Source: CAD feature listing. Evaluate the final solid. Frame: model axes, mm. Face numbers are marked on the shaded views. A direction names the side the tool comes from. Give positions to 0.01 mm unless a question says otherwise; leave off trailing zeros. Order: outer loops, then holes, each group sorted by start corner. A loop starts at its lowest first (then second) coordinate and runs counter-clockwise, first axis right, second up. Notation, with made-up numbers: (36.25, 49) - (50.25, 49) arc R23 cw to (50.25, 82) - close; hole circle Ø6 at (75, -37). An arc over 180 degrees is marked (long way). Use CSV: the item, a comma, the result in double quotes.
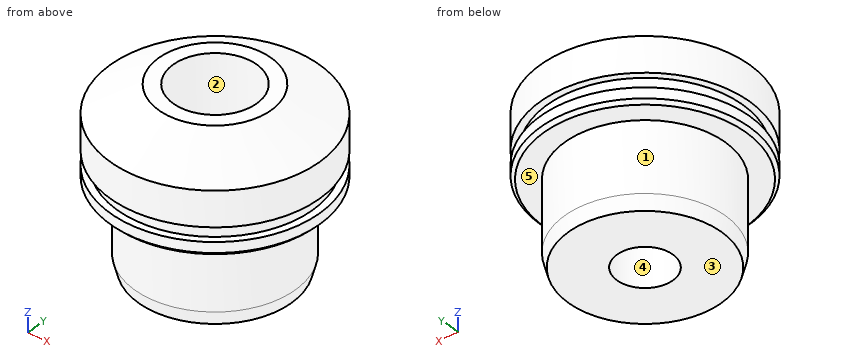
```python
from build123d import *

# Parameters (mm, degrees)
F2_SIZE2 = 0.535898
F2_SIZE  = 2
F3_SIZE  = 0.5


with BuildPart() as f1:
    # F0 (on Front) → F1 (revolve)
    with BuildSketch(Plane.XZ):
        Polygon((-6, 15), (-6, 25), (-8.071797, 25), (-15, 21), (-15, 16), (-14, 16), (-14, 14), (-15, 14), (-15, 12), (-11.5, 12), (-11.5, 0), (-4, 0), (-4, 15), align=None)
    revolve(axis=Axis((0, 0, 15.110009), (0, 0, 1)))

    # F2
    f2_edges = [f1.edges().sort_by_distance(p)[0] for p in [
        (11.5, 0, 0),
    ]]
    chamfer(f2_edges, length=F2_SIZE, length2=F2_SIZE2)

    # F3
    f3_edges = [f1.edges().sort_by_distance(p)[0] for p in [
        (15, 0, 12),
    ]]
    chamfer(f3_edges, length=F3_SIZE)


solid = f1.part
```
Item 1: Set-up query: the marked faces 4 and 5. Return all of +Z, -Z, +X, -X, +Y, -Y with unobstructed straight access to the full face (end or side cutting, diameter ignored); none if empty.
Filled in:
face 4,"+Z, -Z"
face 5,"-Z"
Item 2: Section C-C on z = 6.5. Return the cut outline in (x, y).
Filled in:
outline,"circle Ø23 at (0, 0); hole circle Ø8 at (0, 0)"
Item 3: Mould query, pull axis X, two halves, no side actions, for the marked faces 1, 2 and 3. Classes: released by +X, released by -X, zero draft, split by the parting line, or undercut.
Filled in:
face 1,"split by the parting line"
face 2,"undercut"
face 3,"zero draft"
Item 4: First-contact query: pin 1 (6 mm diameter, centred on y = -5, z = 14, fed in from -X); pin 2 (12 mm diameter, centred on y = -9, z = 5, fed in from +X); pin 3 (5 mm diameter, centred on x = 5.5, z = 8.5, fed in from -Y). Flat tips, straight axial feed; report the tip coordinate or a pass-through.
Filled in:
pin 1,"stops at x = -14.87"
pin 2,"stops at x = 11.1"
pin 3,"stops at y = -11.1"
Item 5: Section D-D on z = 15.5. Return the cut outline in (x, y).
Filled in:
outline,"circle Ø28 at (0, 0); hole circle Ø12 at (0, 0)"
Item 6: Material intervals for line 1 (Y direction, x = 0, z = 6.5); line 2 (Z direction, x = -11.25, y = 9.5), sorted ascending. Write a range as from..to.
Filled in:
line 1,"y = -11.5..-4, 4..11.5"
line 2,"z = 12.22..14, 16..21.16"
